from build123d import *

# Parameters (mm, degrees)
F0_W     = 235
F0_H     = 190
F1_DEPTH = 1
F2_W     = 235
F2_H     = 1
F3_DEPTH = 58
F4_R     = 1.5
F5_DEPTH = 192.001
F6_R     = 0.5
F7_R     = 1


with BuildPart() as f1:
    # F0 (on Top) → F1 (new body)
    with BuildSketch(Plane.XY):
        Rectangle(F0_W, F0_H)
    extrude(amount=F1_DEPTH)

    # F2 (on face) → F3 (join)
    with BuildSketch(Plane.XY.offset(1)):
        with Locations((0, -95.5)):
            Rectangle(F2_W, F2_H)
        with Locations((0, 95.5)):
            Rectangle(F2_W, F2_H)
    extrude(amount=-F3_DEPTH)

    # F4 (on face) → F5 (cut, through all)
    with BuildSketch(Plane.XZ.offset(96)):
        with Locations((-104, -50)):
            Circle(F4_R)
        with Locations((104, -50)):
            Circle(F4_R)
    extrude(amount=-F5_DEPTH, mode=Mode.SUBTRACT)

    # F6
    f6_edges = [f1.edges().sort_by_distance(p)[0] for p in [
        (0, -96, 1),
        (0, 96, 1),
        (0, -95, 0),
        (0, 95, 0),
    ]]
    fillet(f6_edges, radius=F6_R)

    # F7
    f7_edges = [f1.edges().sort_by_distance(p)[0] for p in [
        (-117.5, -95.5, -57),
        (117.5, -95.5, -57),
        (117.5, 95.5, -57),
        (-117.5, 95.5, -57),
    ]]
    fillet(f7_edges, radius=F7_R)


solid = f1.part
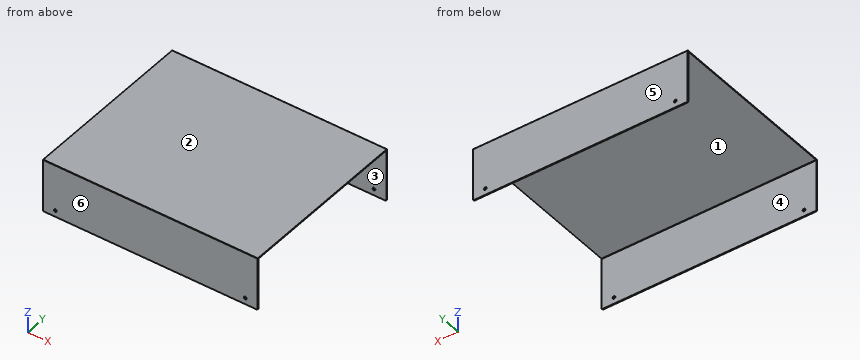
Read the model definition and answer for the solid it produces. Units are mm, in the model's axes. Face numbers are marked on the shaded views. A direction names the side the tool comes from. Round coordinates to 2 decimals unless told otherwise and drop trailing zeros. Write each loop counter-clockwise with the first axis right and the second up, starting at its lowest first coordinate (ties: lowest second). Pieces come first, ordered by that corner, then holes.
1. Determine the mould class of the marked faces 3, 4, 5 and 6 for opening direction Y: pulls with the +Y half, pulls with the -Y half, needs draft (parallel to the pull), parting line crosses it, or undercut.
2. Given pin 1 Ø10 at (x, y) = (-36, -32.5) entering from -Z, flat-ended and moving along its own axis, determine where the tip first touches the part or whether it passes through.
3. The part is cut by section B-B, the plane x = 44.5. Determine the outline of the cut face in (y, z), then the cut area to 3 significant figures.
4. Which of the six approach directions +Z, -Z, +X, -X, +Y, -Y give full straight-line access (tool end or side, diameter ignored) to the marked faces 1 and 2?
5. The part is cut by section A-A, the plane z = -42.5. Determine the outline of the cut face in (x, y), then the cut area to 3 significant figures.
6. Straight lines are drawn through the part: L1, parallel to Y at x = -50.5, z = -12.5; L2, parallel to Z at x = 104, y = 95.45; L3, parallel to Z at x = -4.5, y = -80.5. For each, find the intervals that lie inside material, in ascending order.
7. The part is cut by section C-C, the plane y = 82. Determine the outline of the cut face in (x, z), then the cut area to 3 significant figures.
Values:
1. face 3: undercut
1. face 4: undercut
1. face 5: pulls with the +Y half
1. face 6: pulls with the -Y half
2. pin 1: stops at z = 0
3. outline: (-96, -57) - (-95, -57) - (-95, -0.5) arc R0.5 cw to (-94.5, 0) - (94.5, 0) arc R0.5 cw to (95, -0.5) - (95, -57) - (96, -57) - (96, 0.5) arc R0.5 ccw to (95.5, 1) - (-95.5, 1) arc R0.5 ccw to (-96, 0.5) - close
3. area: 306 mm2
4. face 1: -Z, +X, -X
4. face 2: +Z, +X, -X, +Y, -Y
5. outline: (-117.5, -96) - (117.5, -96) - (117.5, -95) - (-117.5, -95) - close; (-117.5, 95) - (117.5, 95) - (117.5, 96) - (-117.5, 96) - close
5. area: 470 mm2
6. L1: y = -96 to -95, 95 to 96
6. L2: z = -57 to -51.5, -48.5 to 1
6. L3: z = 0 to 1
7. outline: (-117.5, 0) - (117.5, 0) - (117.5, 1) - (-117.5, 1) - close
7. area: 235 mm2
